Geometry: final body of the model. Coordinates: model frame, mm. A direction names the side the tool comes from. Coordinates: 2 decimals unless noted, no trailing zeros. Order: outer loops, then holes, each group sorted by start corner. A loop starts at its lowest first (then second) coordinate and runs counter-clockwise, first axis right, second up. Notation, with made-up numbers: M 18,-13 L 64,-13 A23 ccw 64,25 Z; hole C 16,-13 d11. An arc over 180 degrees is marked long. One line per question, with ' | ' between items.
from build123d import *

# Parameters (mm, degrees)
SKETCH1_R           = 30
SKETCH1_W           = 12.5
SKETCH1_H           = 23.2
BOSS_EXTRUDE1_DEPTH = 5
SKETCH4_R           = 30
SKETCH4_R_2         = 27.5
BOSS_EXTRUDE3_DEPTH = 20
CUT_EXTRUDE2_REACH  = 48.904
SKETCH5_R           = 1.05


with BuildPart() as part:
    # Sketch1 → Boss-Extrude1 (new body)
    with BuildSketch(Plane(origin=(0, 0, 0), x_dir=(1, 0, 0), z_dir=(0, 1, 0))):
        with Locations(Location((0, 0, 0), (0, 0, 270))):
            Circle(SKETCH1_R)
        with Locations((0, 4.1)):
            Rectangle(SKETCH1_W, SKETCH1_H, mode=Mode.SUBTRACT)
    extrude(amount=BOSS_EXTRUDE1_DEPTH)

    # Sketch4 → Boss-Extrude3 (add)
    with BuildSketch(Plane(origin=(0, 5, 0), x_dir=(1, 0, 0), z_dir=(0, 1, 0))):
        with Locations(Location((0, 0, 0), (0, 0, 270))):
            Circle(SKETCH4_R)
        with Locations(Location((0, 0, 0), (0, 0, 270))):
            Circle(SKETCH4_R_2, mode=Mode.SUBTRACT)
    extrude(amount=BOSS_EXTRUDE3_DEPTH)

    # Sketch5 → Cut-Extrude2 (cut, up to next)
    with BuildSketch(Plane(origin=(0, 5, 0), x_dir=(1, 0, 0), z_dir=(0, 1, 0)), mode=Mode.PRIVATE) as cut_extrude2_sk1:
        with Locations(Location((0, 18.2, 0), (0, 0, 270))):
            Circle(SKETCH5_R)
    cut_extrude2_tool1 = extrude(cut_extrude2_sk1.sketch, amount=-CUT_EXTRUDE2_REACH, mode=Mode.PRIVATE) & part.part
    # Sketch5 → Cut-Extrude2 (cut, up to next)
    with BuildSketch(Plane(origin=(0, 5, 0), x_dir=(1, 0, 0), z_dir=(0, 1, 0)), mode=Mode.PRIVATE) as cut_extrude2_sk2:
        with Locations(Location((0, -10, 0), (0, 0, 270))):
            Circle(SKETCH5_R)
    cut_extrude2_tool2 = extrude(cut_extrude2_sk2.sketch, amount=-CUT_EXTRUDE2_REACH, mode=Mode.PRIVATE) & part.part
    add(cut_extrude2_tool1.solids().sort_by_distance((0, 5, -18.2))[0], mode=Mode.SUBTRACT)
    add(cut_extrude2_tool2.solids().sort_by_distance((0, 5, 10))[0], mode=Mode.SUBTRACT)


solid = part.part
1. Section C-C, the plane x = -5.5. Output: boundary loops of the cut face in (y, z).
Response values:
outline: M 0,-29.49 L 25,-29.49 L 25,-26.94 L 5,-26.94 L 5,-15.7 L 0,-15.7 Z; M 0,7.5 L 5,7.5 L 5,26.94 L 25,26.94 L 25,29.49 L 0,29.49 Z
2. Pin query (flat end, axial travel): P1, Ø5, axis at x = -13, y = 20, coming from the -Z side; P2, Ø4, axis at y = 3, z = -5, coming from the -X side; P3, Ø1.5, axis at y = 12.5, z = -18, coming from the -X side. Return the tip coordinate at first contact, or that it passes through.
Response values:
P1: stops at z = -28.1 | P2: stops at x = -29.85 | P3: stops at x = -24.54
3. Material intervals for line 1 (Y direction, x = -24, z = 1); line 2 (Z direction, x = 5.5, y = 1); line 3 (Z direction, x = -18, y = 22.5), sorted ascending. Write a range as [from, to].
Response values:
line 1: y = [0, 5] | line 2: z = [-29.49, -15.7], [7.5, 29.49] | line 3: z = [-24, -20.79], [20.79, 24]
4. Section A-A, the plane z = 0. Output: boundary loops of the cut face in (x, y), and give its area (4 significant figures).
Response values:
outline: M -30,0 L -6.25,0 L -6.25,5 L -27.5,5 L -27.5,25 L -30,25 Z; M 6.25,0 L 30,0 L 30,25 L 27.5,25 L 27.5,5 L 6.25,5 Z | area: 337.5 mm^2
5. Draft query along Z for faces 1 (the face through (1.32, 12.32, -29.97)), 2 (the face through (7, 0, 0)), 3 (the face through (-24.397, 14.86, 12.69)). Return one class per face: pulls with the +Z half, pulls with the -Z half, needs draft (parallel to the pull), parting line crosses it, or undercut.
Response values:
face 1: parting line crosses it | face 2: needs draft | face 3: undercut
6. Section B-B, the plane y = 2.5. Output: boundary loops of the cut face in (x, z).
Response values:
outline: C 0,0 d60; hole M -6.25,-15.7 L 6.25,-15.7 L 6.25,7.5 L -6.25,7.5 Z; hole C 0,-18.2 d2.1; hole C 0,10 d2.1
7. Section D-D, the plane x = -24. Output: boundary loops of the cut face in (y, z).
Response values:
outline: M 0,-18 L 25,-18 L 25,-13.43 L 5,-13.43 L 5,13.43 L 25,13.43 L 25,18 L 0,18 Z
8. Access query for faces 4 (the face through (0, 2, -15.7)), 5 (the face through (6.5, 5, -0.4)), 6 (the face through (-24.3, 25, 13.2)). Directions: +Z, -Z, +X, -X, +Y, -Y. A direction counts if a zero-diameter tool reaches every point of the face in a straight line with its end or side. Return the directions, or none.
Response values:
face 4: +Y, -Y | face 5: +Y | face 6: +Z, -Z, +X, -X, +Y
